Design review of the part built by this model. Coordinates are the model's own, in mm. A direction names the side the tool comes from. Coordinates: 2 decimals unless noted, no trailing zeros. Loops run counter-clockwise (first coordinate to the right, second up) from the corner with the lowest first, then second, coordinate; pieces in that order, holes last. Notation, with made-up numbers: (78.25, -35) - (94.25, -35) arc R32 ccw to (94.25, -6) - close; hole circle Ø7 at (11, -0.75). An arc over 180 degrees is marked (long way). Answer in a Markdown table with one row per item. Add a question column.
(1) Clearance check with flat-ended pins moving along their axes: pin 1 (1.5 mm diameter, centred on x = 9, z = 17, fed in from -Y); pin 2 (1.5 mm diameter, centred on x = -3, y = 4, fed in from -Z); pin 3 (6 mm diameter, centred on x = -11, z = 43.5, fed in from -Y); pin 4 (8 mm diameter, centred on x = -20, z = 14.5, fed in from -Y). State where each tip first meets the part, or that it passes through.
(2) We need section C-C, the plane y = 18. Write out the cut boundary in (x, z).
(3) For faces 5 (the face through (12.169, 29.094, 0.811)), 6 (the face through (0, 25, 1.6)), list the 3-axis set-ups (+Z, -Z, +X, -X, +Y, -Y) from which the entire face can be reached by the end or side of a thin tool; tool diameter is ignored.
(4) To check wall thickness, follow L1, parallel to X at y = 4, z = 1; L2, parallel to Y at x = -13, z = 1.05; L3, parallel to Y at x = 13, z = 1. State the ranges of each line that lie inside material, in increasing order. Write a range as [from, to].
(5) We need section A-A, the plane y = 4. Write out the cut boundary in (x, z).
(6) We need section D-D, the plane z = 9.5. Write out the cut boundary in (x, y).
(7) The part is to be moulded in two halves that separate along Z. For faces 1 (the face through (-23.4, -34.99, 48.97)), 2 (the face through (-4.054, -33.425, 46.771)), 3 (the face through (-1.08, 35.32, 0.81)), 4 (the face through (-19.054, -33.425, 46.771)), say which applies: released by +Z, released by -Z, zero draft, split by the parting line, or undercut.
(8) We need section B-B, the plane x = 0. Write out the cut boundary in (y, z) (3 decimals), plus the area to 3 significant figures.
Autodesk Inventor part; units mm, degrees
ref_plane "YZ Plane" through (0, 0, 0) normal (1, 0, 0) x (0, 1, 0)
ref_plane "XZ Plane" through (0, 0, 0) normal (0, 1, 0) x (-1, 0, 0)
ref_plane "XY Plane" through (0, 0, 0) normal (0, 0, 1) x (1, 0, 0)
sketch "スケッチ1" plane through (0, 0, 0) normal (0, 0, 1) x (1, 0, 0)
  line L0 (20, 0) -> (-20, 0)
  line L1 (-20, 0) -> (-20, 50)
  line L2 (-20, 50) -> (20, 50)
  line L3 (20, 50) -> (20, 0)
  line L4 (20, 0) -> (-20, 50) construction
  line L5 (-20, 0) -> (20, 50) construction
  point P0 (0, 0)
  point P1 (0, 25)
  point P2 (0, 0)
  point P3 (0, 25)
  dimension "d0" = 40
  dimension "d1" = 50
extrude "プレート1" add sketch "スケッチ1" along normal blind 1.6
sketch "スケッチ2" plane through (20, -1.3106, 2.2823) normal (0, -0.819152, -0.5735764) x (1, 0, 0)
  line L0 (-40, 0) -> (0, 0)
  line L1 (0, 0) -> (0, 58.1342)
  line L2 (0, 58.1342) -> (-40, 58.1342)
  line L3 (-40, 58.1342) -> (-40, 0)
edge flange "フランジ1" height 59.8 angle 55 thickness 1.6 bend radius 1.6 thickness toward (0, -0.819152, -0.5735764) relief tear relief width 1.6 relief depth 0.8 edges at (0, 0, 1.6) wall of the first edge with corners at (-20, -1.3106, 2.2823) (20, -1.3106, 2.2823) (20, -34.655, 49.903) (-20, -34.655, 49.903)
bend "曲げ1"
corner "コーナー1"
sketch "スケッチ3" plane through (0, 0, 0) normal (0, 0, -1) x (-1, 0, 0)
  line L0 (-20, 0) -> (20, 0)
  line L1 (20, 0) -> (20, 50)
  line L2 (20, 50) -> (-20, 50)
  line L3 (-20, 50) -> (-20, 0)
  line L4 (-20, 0) -> (20, 0)
  point P0 (0, 0)
  point P1 (-13, 4)
  point P2 (13, 4)
  point P3 (0, 4)
  point P4 (0, 0)
  point P5 (0, 0)
  point P6 (0, 4)
  point P7 (-13, 30)
  point P8 (13, 30)
  dimension "d62" = 4
  dimension "d85" = 26
  dimension "d86" = 13
  dimension "d90" = 26
hole "穴1" at (13, 4, 0) at (-13, 4, 0) at (13, 30, 0) at (-13, 30, 0) direction (0, 0, 1) diameter 2.459 depth 8.8 tip angle 118
sketch "スケッチ4" plane through (-20, -35.9657, 48.9853) normal (0, -0.819152, -0.5735764) x (1, 0, 0)
  line L0 (0, -58.1342) -> (40, -58.1342)
  line L1 (40, 0) -> (40, -58.1342)
  line L2 (0, 0) -> (40, 0)
  line L3 (0, -58.1342) -> (0, 0)
  point P0 (20, -60.7555)
  point P1 (35, -54.1342)
  dimension "d23" = 5
  dimension "d24" = 4
hole "穴2" at (15, -4.9156, 4.6412) direction (0, 0.819152, 0.5735764) diameter 2.459 end through all
sketch "スケッチ5" plane through (-20, -35.9657, 48.9853) normal (0, -0.819152, -0.5735764) x (1, 0, 0)
  circle A0 centre (35, -54.1342) radius 1.2295
  line L0 (0, 0) -> (0, -58.1342)
  line L1 (0, -12.1342) -> (-12, -12.1342)
  line L2 (-12, -12.1342) -> (-12, -20.1342)
  line L3 (-12, -20.1342) -> (0, -20.1342)
  line L4 (0, -20.1342) -> (0, -12.1342)
  point P0 (20, -60.7555)
  point P1 (-8, -16.1342)
  point P2 (0, -20.1342)
  dimension "d32" = 43
  dimension "d33" = 38
  dimension "d34" = 4
  dimension "d35" = 8
  dimension "d36" = 4
extrude "押し出し1" add sketch "スケッチ5" against normal up to surface (1.6 mm away) contours L0 L3 L2 L1
sketch "スケッチ6" plane through (-20, -35.9657, 48.9853) normal (0, -0.819152, -0.5735764) x (1, 0, 0)
  circle A0 centre (35, -54.1342) radius 1.2295
  point P0 (20, -60.7555)
  point P1 (-8, -16.1342)
  dimension "d39" = 43
  dimension "d40" = 38
hole "穴3" at (-28, -26.7115, 35.7689) direction (0, 0.819152, 0.5735764) diameter 2.459 depth 8.8 tip angle 118
fillet "フィレット1" radius 4 2 edges at (-32, -23.7619, 32.9512) (-32, -28.3505, 39.5044)
fillet "フィレット2" radius 2 2 edges at (20, 50, 0.8) (-20, 50, 0.8)
sketch "スケッチ8" plane through (-20, -35.9657, 48.9853) normal (0, -0.819152, -0.5735764) x (1, 0, 0)
  line L0 (0, 0) -> (0, -12.1342)
  line L1 (0, 0) -> (-1, 0)
  line L2 (-1, 0) -> (-1, -12.1342)
  line L3 (-1, -12.1342) -> (0, -12.1342)
  line L4 (0, -12.1342) -> (0, 0)
  point P0 (20, -60.7555)
  point P1 (0, -12.1342)
  dimension "d63" = 1
extrude "押し出し3" add sketch "スケッチ8" against normal up to surface (1.6 mm away)
sketch "スケッチ9" plane through (-20, -2.6213, 1.3646) normal (0, -0.819152, -0.5735764) x (1, 0, 0)
  line L0 (40, 58.1342) -> (-1, 58.1342)
  line L1 (-1, 58.1342) -> (-1, 46)
  point P0 (20, -2.6213)
  point P1 (1, 53.6342)
  point P2 (16, 53.6342)
  dimension "d66" = 4.5
  dimension "d67" = 15
  dimension "d68" = 2
hole "穴4" at (-19, -33.3846, 45.2991) at (-4, -33.3846, 45.2991) direction (0, 0.819152, 0.5735764) diameter 2.459 end through all
sketch "スケッチ10" plane through (-20, -2.6213, 1.3646) normal (0, -0.819152, -0.5735764) x (1, 0, 0)
  line L0 (43, 58.1342) -> (-4, 58.1342)
  line L1 (-4, 58.1342) -> (-4, 50.1342)
  line L2 (-4, 50.1342) -> (43, 50.1342)
  line L3 (43, 50.1342) -> (43, 58.1342)
  line L4 (-1, 58.1342) -> (-1, 46)
  line L5 (40, 58.1342) -> (40, 0)
  line L6 (-1, 46) -> (-8, 46)
  line L7 (-4, 50.1342) -> (-1, 50.1342)
  line L8 (-1, 50.1342) -> (-1, 46)
  line L9 (-1, 46) -> (-4, 46)
  line L10 (-4, 46) -> (-4, 50.1342)
  point P0 (20, -2.6213)
  point P1 (-4, 46)
  dimension "d76" = 3
  dimension "d77" = 3
  dimension "d78" = 8
extrude "押し出し4" add sketch "スケッチ10" against normal up to surface (1.6 mm away) contours L4 L2 L1 L0 | L4 L6 L10 L2
chamfer "面取り4" distance 2 angle 45 2 edges at (-20, -23.7619, 32.9512) (-24, -28.3505, 39.5044)
fillet "フィレット3" radius 2 6 edges at (-20, -22.6147, 31.3129) (-22, -23.7619, 32.9512) (-26, -28.3505, 39.5044) (-24, -29.4976, 41.1427) (-24, -35.3104, 49.4442) (20, -35.3104, 49.4442)
sketch "スケッチ12" plane through (0, 0, 0) normal (0, 0, -1) x (-1, 0, 0)
  line L0 (-15, 36.5) -> (15, 36.5)
  line L1 (15, 36.5) -> (15, 8.5)
  line L2 (15, 8.5) -> (-15, 8.5)
  line L3 (-15, 8.5) -> (-15, 36.5)
  line L4 (-20, 0) -> (20, 0)
  point P0 (0, 0)
  point P1 (0, 36.5)
  dimension "d91" = 28
  dimension "d92" = 30
  dimension "d93" = 15
  dimension "d94" = 8.5
hole "穴5" at (15, 8.5, 0) at (-15, 8.5, 0) at (0, 36.5, 0) direction (0, 0, 1) diameter 3.2 depth 1.6 tip angle 118
equation "\"d30\" = Thickness"
equation "\"d100\" = Thickness"
equation "\"d2\" = Thickness"
equation "\"d3\" = BendReliefWidth"
equation "\"d4\" = BendReliefDepth"
equation "\"d5\" = MinimumRemnant"
equation "\"d6\" = TransitionRadius"
equation "\"d9\" = BendRadius"
equation "\"d10\" = CornerReliefSize"
equation "\"d11\" = GapSize"
equation "\"d12\" = JacobiRadiusSize"
equation "\"BendRadius\" = Thickness"
equation "\"BendReliefWidth\" = Thickness"
equation "\"BendReliefDepth\" = 0.5 * Thickness"
equation "\"CornerReliefSize\" = 4 * Thickness"
equation "\"MinimumRemnant\" = 2 * Thickness"
equation "\"TransitionRadius\" = BendRadius"
equation "\"JacobiRadiusSize\" = BendRadius"
equation "\"GapSize\" = Thickness"
properties part number "Fan_Holder"
Responses:
| question | item | result |
|---|---|---|
| 1 | pin 1 | stops at y = -14.09 |
| 1 | pin 2 | stops at z = 0 |
| 1 | pin 3 | stops at y = -34.23 |
| 1 | pin 4 | stops at y = -14.62 |
| 2 | outline | (-20, 0) - (20, 0) - (20, 1.6) - (-20, 1.6) - close |
| 3 | face 5 | +Z, -Z |
| 3 | face 6 | +Z, +X, -X, +Y |
| 4 | L1 | x = [-20, -14.23], [-11.77, 11.77], [14.23, 20] |
| 4 | L2 | y = [-2.37, 2.77], [5.23, 28.77], [31.23, 50] |
| 4 | L3 | y = [-2.32, 2.77], [5.23, 28.77], [31.23, 50] |
| 5 | outline | (-20, 0) - (-14.23, 0) - (-14.23, 1.6) - (-20, 1.6) - close; (-11.77, 0) - (11.77, 0) - (11.77, 1.6) - (-11.77, 1.6) - close; (14.23, 0) - (20, 0) - (20, 1.6) - (14.23, 1.6) - close |
| 6 | outline | (-20, -8.32) - (20, -8.32) - (20, -6.36) - (-20, -6.36) - close |
| 7 | face 1 | released by +Z |
| 7 | face 2 | undercut |
| 7 | face 3 | zero draft |
| 7 | face 4 | undercut |
| 8 | outline | (-35.966, 48.985) - (-2.621, 1.365) arc R3.2 ccw to (0, 0) - (34.9, 0) - (34.9, 1.6) - (0, 1.6) arc R1.6 cw to (-1.311, 2.282) - (-34.655, 49.903) - close; (38.1, 0) - (50, 0) - (50, 1.6) - (38.1, 1.6) - close |
| 8 | area | 172 mm2 |
